Read the model definition and answer for the solid it produces. Units are mm, in the model's axes. A direction names the side the tool comes from. Round coordinates to 2 decimals unless told otherwise and drop trailing zeros. Order: outer loops, then holes, each group sorted by start corner. A loop starts at its lowest first (then second) coordinate and runs counter-clockwise, first axis right, second up. Notation, with made-up numbers: (85.25, 44) - (107.25, 44) arc R22 ccw to (107.25, 76) - close; hole circle Ø8 at (7, -28). An arc over 180 degrees is marked (long way). One line per question, with ' | ' between items. Start each with the question number.
1) Straight lines are drawn through the part: line 1 (X direction, y = -7.25, z = 0.6); line 2 (X direction, y = -11.5, z = 0.25); line 3 (X direction, y = -9.25, z = 0.9). For each, find the intervals that lie inside material, in ascending order. Write a range as from..to.
2) The mould has two halves that part along X. Classify faces 3 (the flat face through (-0.4, 12.5, 0.5)), 4 (the flat face through (25.4, -0.2, 0.5)), 5 (the flat face through (-12.12, -8.9, 0.51)): pulls with the +X half, pulls with the -X half, needs draft (parallel to the pull), parting line crosses it, or undercut.
3) The part is cut by section B-B, the plane z = 0.8. Give the vertices of the cut face in (x, y).
4) The part is cut by section A-A, the plane y = -9. Give the vertices of the cut face in (x, z), plus the area to 3 significant figures.
5) Flat-ended cylindrical pins translate along their axes: pin 1 (12 mm diameter, centred on x = -5.5, y = 8, fed in from -Z); pin 2 (1.8 mm diameter, centred on x = 18.55, y = -8.08, fed in from +Z). Find the tip coordinate at first contact, or state that the pin passes through.
6) For faces 1 (the flat face through (-15.715, -8.797, 0.507)), 2 (the flat face through (-25.4, -0.2, 0.5)), determine the directions among +Z, -Z, +X, -X, +Y, -Y from which every point of the face is accessible in a straight line to the end or side of a thin tool.
from build123d import *

# Parameters (mm, degrees)
F0_W     = 50.8
F0_H     = 25
F1_DEPTH = 1
F2_R     = 1.5
F3_DEPTH = 25
F5_DEPTH = 25


with BuildPart() as f1:
    # F0 (on Top) → F1 (new body)
    with BuildSketch(Plane.XY):
        Rectangle(F0_W, F0_H)
    extrude(amount=F1_DEPTH)

    # F2 (on face) → F3 (cut)
    with BuildSketch(Plane.XY.offset(1)):
        with Locations((18.549042, -8.076559)):
            Circle(F2_R)
    extrude(amount=-F3_DEPTH, mode=Mode.SUBTRACT)

    # F4 (on face) → F5 (cut)
    with BuildSketch(Plane.XY.offset(1)):
        Polygon((-15.12827, -5.19568), (-16.317381, -12.5), (-9.196741, -12.5), align=None)
    extrude(amount=-F5_DEPTH, mode=Mode.SUBTRACT)


solid = f1.part
Values:
1) line 1: x = -25.4..-15.46, -13.46..17.3, 19.8..25.4 | line 2: x = -25.4..-16.15, -10.01..25.4 | line 3: x = -25.4..-15.79, -11.84..17.61, 19.48..25.4
2) face 3: needs draft | face 4: pulls with the +X half | face 5: undercut
3) outline: (-25.4, -12.5) - (-16.32, -12.5) - (-15.13, -5.2) - (-9.2, -12.5) - (25.4, -12.5) - (25.4, 12.5) - (-25.4, 12.5) - close; hole circle Ø3 at (18.55, -8.08)
4) outline: (-25.4, 0) - (-15.75, 0) - (-15.75, 1) - (-25.4, 1) - close; (-12.04, 0) - (17.37, 0) - (17.37, 1) - (-12.04, 1) - close; (19.73, 0) - (25.4, 0) - (25.4, 1) - (19.73, 1) - close | area: 44.7 mm^2
5) pin 1: stops at z = 0 | pin 2: passes through
6) face 1: +Z, -Z, -Y | face 2: +Z, -Z, -X, +Y, -Y
